Source: three-view drawing plus pictorial views. Frame: mm from the lowest corner of the part. A direction names the side the tool comes from. Round coordinates to 2 decimals unless told otherwise and drop trailing zeros. Write each loop counter-clockwise with the first axis right and the second up, starting at its lowest first coordinate (ties: lowest second). Pieces come first, ordered by that corner, then holes.
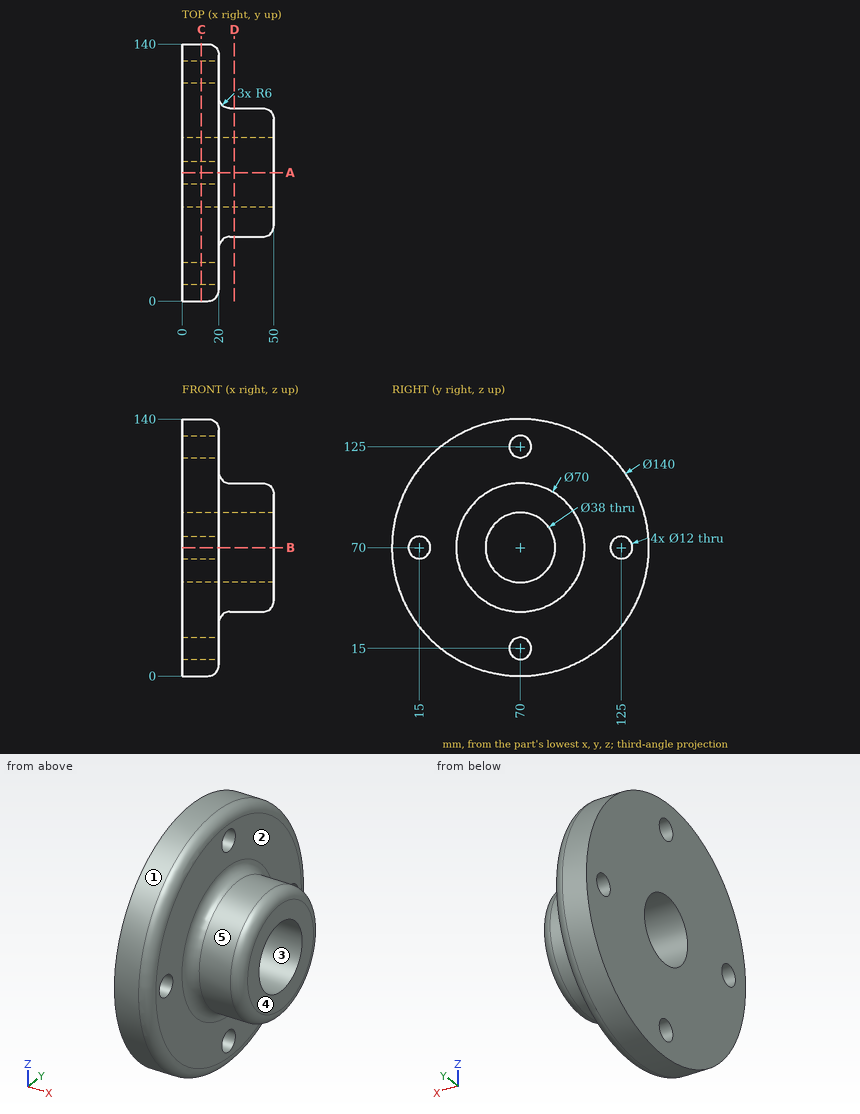
1) Draft query along Y for the marked faces 1, 2 and 3. Return one class per face: pulls with the +Y half, pulls with the -Y half, needs draft (parallel to the pull), parting line crosses it, or undercut.
2) Section D-D on x = 28.5. Output: boundary loops of the cut face in (y, z).
3) Line query: probe 1 along Y at (x, z) = (9.75, 70); probe 2 along Y at (x, z) = (37.5, 70); probe 3 along X at (y, z) = (77.5, 131.5). Output: solid intervals per line, ascending.
4) First-contact query: P1, Ø19, axis at y = 70, z = 15, coming from the +X side; P2, Ø10, axis at x = 14, z = 109, coming from the -Y side; P3, Ø1, axis at x = 12.5, z = 48, coming from the +Y side; P4, Ø7, axis at y = 70, z = 125, coming from the -X side. Flat tips, straight axial feed; report the tip coordinate or a pass-through.
5) Section C-C on x = 10.5. Output: boundary loops of the cut face in (y, z).
6) Reachability of the marked faces 4 and 5 from +Z, -Z, +X, -X, +Y, -Y: full face, straight path, thin tool, end or side. Return the list, or none.
7) Section A-A on y = 70. Output: boundary loops of the cut face in (x, z).
Filled in:
1. face 1: parting line crosses it
1. face 2: needs draft
1. face 3: undercut
2. outline: circle Ø70 at (70, 70); hole circle Ø38 at (70, 70)
3. probe 1: y = 0 to 9, 21 to 51, 89 to 119, 131 to 140
3. probe 2: y = 35 to 51, 89 to 105
3. probe 3: x = 0 to 20
4. P1: stops at x = 20
4. P2: stops at y = 8.81
4. P3: stops at y = 136.62
4. P4: passes through
5. outline: circle Ø140 at (70, 70); hole circle Ø12 at (15, 70); hole circle Ø38 at (70, 70); hole circle Ø12 at (70, 15); hole circle Ø12 at (70, 125); hole circle Ø12 at (125, 70)
6. face 4: +Z, -Z, +X, +Y, -Y
6. face 5: +X
7. outline: (0, 0) - (14, 0) arc R6 ccw to (20, 6) - (20, 9) - (0, 9) - close; (0, 21) - (20, 21) - (20, 29) arc R6 cw to (26, 35) - (44, 35) arc R6 ccw to (50, 41) - (50, 51) - (0, 51) - close; (0, 89) - (50, 89) - (50, 99) arc R6 ccw to (44, 105) - (26, 105) arc R6 cw to (20, 111) - (20, 119) - (0, 119) - close; (0, 131) - (20, 131) - (20, 134) arc R6 ccw to (14, 140) - (0, 140) - close
